The listing builds one solid part. Answer for the finished solid, in the listing's coordinates (mm). Face numbers are marked on the shaded views. A direction names the side the tool comes from. Coordinates: 2 decimals unless noted, no trailing zeros. Loops run counter-clockwise (first coordinate to the right, second up) from the corner with the lowest first, then second, coordinate; pieces in that order, holes last. Notation, with made-up numbers: M -38,-35 L 8,-35 A20 ccw 8,-16 Z; hole C 60.5,41.25 d9. An arc over 180 degrees is marked long. Return JSON: item names as keys, results as strings. Group by question number.
1. Which of the six approach directions +Z, -Z, +X, -X, +Y, -Y give full straight-line access (tool end or side, diameter ignored) to the marked faces 4, 5, 6, 7 and 8?
2. Straight lines are drawn through the part: L1, parallel to Z at x = -5.25, y = 96; L2, parallel to X at y = 10.5, z = 14.5; L3, parallel to X at y = 69, z = -28. For each, find the intervals that lie inside material, in ascending order. Write a range as from..to.
3. Section C-C (x = -0.5) is taken. Write down the section's boundary in (y, z).
4. Given P1, Ø6, axis at y = 125.5, z = -16.5, coming from the -X side; P2, Ø13, axis at x = -0.5, z = -39.5, coming from the -Y side; P3, Ø8, axis at x = -0.5, z = 28, coming from the -Y side; P4, Ø7, axis at y = 74, z = 10.5, coming from the -X side, each flat-ended and moving along its own axis, determine where each tip first touches the part or whether it passes through.
5. The mould has two halves that part along Z. Classify the marked faces 1, 2 and 3: pulls with the +Z half, pulls with the -Z half, needs draft (parallel to the pull), parting line crosses it, or undercut.
```python
from build123d import *

# Parameters (mm, degrees)
BOSS_EXTRUDE1_DEPTH      = 5
BOSS_EXTRUDE1_2_DEPTH    = 5
BOSS_EXTRUDE1_3_DEPTH    = 5
BOSS_EXTRUDE1_4_DEPTH    = 5
SKETCH5_W                = 5
SKETCH5_H                = 65
BOSS_EXTRUDE6_DEPTH      = 150
SKETCH6_W                = 5
SKETCH6_H                = 125
BOSS_EXTRUDE7_DEPTH      = 12
SKETCH9_W                = 26
SKETCH9_H                = 125
BOSS_EXTRUDE9_DEPTH      = 5
SKETCH7_W                = 26
SKETCH7_H                = 115
BOSS_EXTRUDE8_DEPTH      = 5
CHAMFER1_SIZE            = 10
CHAMFER1_SIZE2           = 5
CHAMFER2_SIZE2           = 10
CHAMFER2_SIZE            = 5
FILLET1_R                = 3
CUT_EXTRUDE2_DEPTH       = 2.5
CUT_EXTRUDE3_DEPTH       = 2.5
CHAMFER3_SIZE            = 2.5
CHAMFER3_OF_MIRROR1_SIZE = 2.5


with BuildPart() as part:
    # Sketch1 → Boss-Extrude1 (new body)
    with BuildSketch(Plane(origin=(0, 0, 0), x_dir=(1, 0, 0), z_dir=(0, 1, 0))):
        Polygon((-13, 19.75), (-13, 12.75), (-8, 11.25), (-8, 21.25), align=None)
    extrude(amount=-BOSS_EXTRUDE1_DEPTH)



with BuildPart() as body_2:
    # Sketch1 → Boss-Extrude1 2 (new body)
    with BuildSketch(Plane(origin=(0, 0, 0), x_dir=(1, 0, 0), z_dir=(0, 1, 0))):
        Polygon((-13, -19.75), (-8, -21.25), (-8, -11.25), (-13, -12.75), align=None)
    extrude(amount=-BOSS_EXTRUDE1_2_DEPTH)


with BuildPart() as body_3:
    # Sketch1 → Boss-Extrude1 3 (new body)
    with BuildSketch(Plane(origin=(0, 0, 0), x_dir=(1, 0, 0), z_dir=(0, 1, 0))):
        Polygon((13, 19.75), (8, 21.25), (8, 11.25), (13, 12.75), align=None)
    extrude(amount=-BOSS_EXTRUDE1_3_DEPTH)


with BuildPart() as body_4:
    # Sketch1 → Boss-Extrude1 4 (new body)
    with BuildSketch(Plane(origin=(0, 0, 0), x_dir=(1, 0, 0), z_dir=(0, 1, 0))):
        Polygon((13, -19.75), (13, -12.75), (8, -11.25), (8, -21.25), align=None)
    extrude(amount=-BOSS_EXTRUDE1_4_DEPTH)


with BuildPart() as part_1:
    add(part.part)

    add(body_2.part)  # Boss-Extrude6 merges body 2

    add(body_3.part)  # Boss-Extrude6 merges body 3

    add(body_4.part)  # Boss-Extrude6 merges body 4
    # Sketch5 → Boss-Extrude6 (add)
    with BuildSketch(Plane(origin=(0, 0, 0), x_dir=(1, 0, 0), z_dir=(0, 1, 0))):
        with Locations((-10.5, 0)):
            Rectangle(SKETCH5_W, SKETCH5_H)
        with Locations((10.5, 0)):
            Rectangle(SKETCH5_W, SKETCH5_H)
    extrude(amount=BOSS_EXTRUDE6_DEPTH)

    # Sketch6 → Boss-Extrude7 (add)
    with BuildSketch(Plane(origin=(0, 0, -32.5), x_dir=(-1, 0, 0), z_dir=(0, 0, -1))):
        with Locations((-10.5, 87.5)):
            Rectangle(SKETCH6_W, SKETCH6_H)
        with Locations((10.5, 87.5)):
            Rectangle(SKETCH6_W, SKETCH6_H)
    extrude(amount=BOSS_EXTRUDE7_DEPTH)

    # Sketch9 → Boss-Extrude9 (add)
    with BuildSketch(Plane(origin=(0, 0, -44.5), x_dir=(-1, 0, 0), z_dir=(0, 0, -1))):
        with Locations((0, 87.5)):
            Rectangle(SKETCH9_W, SKETCH9_H)
    extrude(amount=BOSS_EXTRUDE9_DEPTH)

    # Sketch7 → Boss-Extrude8 (add)
    with BuildSketch(Plane.XY.offset(32.5)):
        with Locations((0, 92.5)):
            Rectangle(SKETCH7_W, SKETCH7_H)
    extrude(amount=BOSS_EXTRUDE8_DEPTH)

    # Chamfer1
    chamfer1_edges = [part_1.edges().sort_by_distance(p)[0] for p in [
        (13, 25, -41),
    ]]
    chamfer1_side = [part_1.faces().sort_by_distance(p)[0] for p in [
        (13, 77.49201278, -5.3514377),
    ]]
    chamfer(chamfer1_edges, length=CHAMFER1_SIZE, length2=CHAMFER1_SIZE2, reference=chamfer1_side[0])

    # Chamfer2
    chamfer2_edges = [part_1.edges().sort_by_distance(p)[0] for p in [
        (-13, 25, -41),
    ]]
    chamfer2_side = [part_1.faces().sort_by_distance(p)[0] for p in [
        (-12.9, 25, -41),
    ]]
    chamfer(chamfer2_edges, length=CHAMFER2_SIZE - 0.0001, length2=CHAMFER2_SIZE2 - 0.0001, reference=chamfer2_side[0])  # a hair under: the kernel refuses the full size

    # Fillet1
    fillet1_edges = [part_1.edges().sort_by_distance(p)[0] for p in [
        (-13, 92.49995, -49.5),
        (13, 92.5, -49.5),
        (13, 92.5, 37.5),
        (-13, 92.5, 37.5),
    ]]
    fillet(fillet1_edges, radius=FILLET1_R)

    # Sketch13 → Cut-Extrude2 (cut)
    with BuildSketch(Plane.ZY.offset(13)):
        Polygon((13.198511713, 150), (4.099255857, 125), (4.099255857, 65), (-5, 40), (-5, 0), (5, 0), (5, 38.236730193), (14.099255857, 63.236730193), (14.099255857, 123.236730193), (23.840289438, 150), align=None)
    cut_extrude2 = extrude(amount=-CUT_EXTRUDE2_DEPTH, mode=Mode.SUBTRACT)

    # Sketch15 → Cut-Extrude3 (cut)
    with BuildSketch(Plane.ZY.offset(13)):
        Polygon((-5.900744143, 66.763269807), (-13.821926553, 45), (-36.5, 45), (-36.5, 140), (-1.082968354, 140), (-5.900744143, 126.763269807), align=None)
    cut_extrude3 = extrude(amount=-CUT_EXTRUDE3_DEPTH, mode=Mode.SUBTRACT)

    # Chamfer3
    chamfer3_edges = [part_1.edges().sort_by_distance(p)[0] for p in [
        (-10.5, 136.618365096, 18.969772647),
        (-10.5, 93.236730193, 14.099255857),
        (-10.5, 50.736730193, 9.549627928),
        (-10.5, 19.118365096, 5),
        (-10.5, 20, -5),
        (-10.5, 52.5, -0.450372072),
        (-10.5, 95, 4.099255857),
        (-10.5, 137.5, 8.648883785),
        (-10.5, 45, -25.160963277),
        (-10.5, 55.881634904, -9.861335348),
        (-10.5, 96.763269807, -5.900744143),
        (-10.5, 133.381634904, -3.491856249),
        (-10.5, 92.5, -36.5),
        (-10.5, 140, -18.791484177),
    ]]
    chamfer(chamfer3_edges, length=CHAMFER3_SIZE - 0.0001)  # a hair under: the kernel refuses the full size

    # Mirror1: Cut-Extrude2, Cut-Extrude3 across plane
    add(cut_extrude2.mirror(Plane(origin=(0, 0, 0), x_dir=(0, 0, 1), z_dir=(1, 0, 0))), mode=Mode.SUBTRACT)
    add(cut_extrude3.mirror(Plane(origin=(0, 0, 0), x_dir=(0, 0, 1), z_dir=(1, 0, 0))), mode=Mode.SUBTRACT)

    # Chamfer3 of Mirror1
    chamfer3_of_mirror1_edges = [part_1.edges().sort_by_distance(p)[0] for p in [
        (10.5, 136.618365096, 18.969772647),
        (10.5, 93.236730193, 14.099255857),
        (10.5, 50.736730193, 9.549627928),
        (10.5, 19.118365096, 5),
        (10.5, 20, -5),
        (10.5, 52.5, -0.450372072),
        (10.5, 95, 4.099255857),
        (10.5, 137.5, 8.648883785),
        (10.5, 45, -25.160963277),
        (10.5, 55.881634904, -9.861335348),
        (10.5, 96.763269807, -5.900744143),
        (10.5, 133.381634904, -3.491856249),
        (10.5, 92.5, -36.5),
        (10.5, 140, -18.791484177),
    ]]
    chamfer(chamfer3_of_mirror1_edges, length=CHAMFER3_OF_MIRROR1_SIZE - 0.0001)  # a hair under: the kernel refuses the full size


solid = part_1.part
```
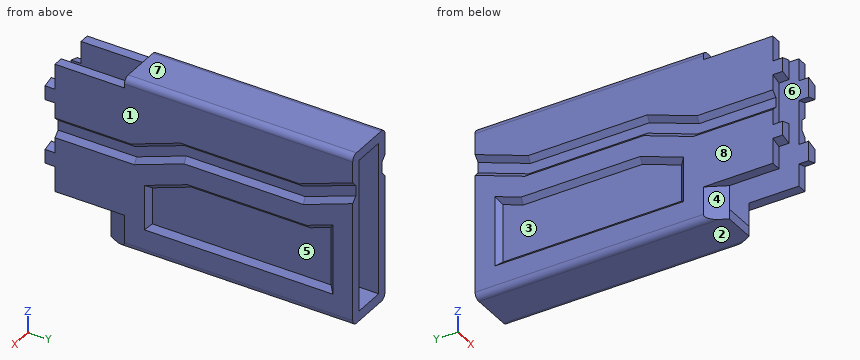
Worked out:
{
 "1": {"face 4": "-Z, -X, -Y", "face 5": "+X", "face 6": "+Y, -Y", "face 7": "+Z, +X, -X, +Y, -Y", "face 8": "+Z, -Z, -X, +Y, -Y"},
 "2": {"L1": "-49.5..-44.5, 32.5..37.5", "L2": "-13..-8, 8..13", "L3": "-10.5..-8, 8..10.5"},
 "3": {"outline": "M 25,-49.5 L 150,-49.5 L 150,-44.5 L 25,-44.5 Z; M 35,32.5 L 150,32.5 L 150,37.5 L 35,37.5 Z"},
 "4": {"P1": "x = -10.5", "P2": "y = 25", "P3": "through", "P4": "x = -12.9"},
 "5": {"face 1": "needs draft", "face 2": "pulls with the -Z half", "face 3": "undercut"}
}
